from build123d import *

# Parameters (mm, degrees)
SKETCH2_W           = 216
SKETCH2_H           = 193.902
SKETCH2_W_2         = 203.3
SKETCH2_H_2         = 181.202
BOSS_EXTRUDE1_DEPTH = 12.7
SKETCH2_3_W         = 203.3
SKETCH2_3_H         = 181.202
BOSS_EXTRUDE2_DEPTH = 6.35
CUT_EXTRUDE1_DEPTH  = 12.7
SKETCH5_W           = 216
SKETCH5_H           = 193.902
CUT_EXTRUDE2_DEPTH  = 1.27


with BuildPart() as part:
    # Sketch2 → Boss-Extrude1 (new body)
    with BuildSketch(Plane(origin=(0, 0, 0), x_dir=(1, 0, 0), z_dir=(0, 1, 0))):
        with Locations((101.6, 90.551)):
            Rectangle(SKETCH2_W, SKETCH2_H)
        with Locations((101.6, 90.551)):
            Rectangle(SKETCH2_W_2, SKETCH2_H_2, mode=Mode.SUBTRACT)
    extrude(amount=BOSS_EXTRUDE1_DEPTH)

    # Sketch2<3> → Boss-Extrude2 (add)
    with BuildSketch(Plane(origin=(0, 0, 0), x_dir=(1, 0, 0), z_dir=(0, 1, 0))):
        with Locations((101.6, 90.551)):
            Rectangle(SKETCH2_3_W, SKETCH2_3_H)
    extrude(amount=BOSS_EXTRUDE2_DEPTH)

    # Sketch4 → Cut-Extrude1 (cut, symmetric)
    with BuildSketch(Plane(origin=(0, 0, -90.551), x_dir=(-1, 0, 0), z_dir=(0, 0, -1))):
        Polygon((-203.2, 9.645710678), (-204.507721606, 8.337989072), (-204.507721606, 7.018410881), (-203.2, 6.26339746), align=None)
    cut_extrude1 = extrude(amount=CUT_EXTRUDE1_DEPTH, both=True, mode=Mode.SUBTRACT)

    # Sketch5 → Cut-Extrude2 (cut)
    with BuildSketch(Plane(origin=(0, 12.7, 0), x_dir=(1, 0, 0), z_dir=(0, 1, 0))):
        with Locations((101.6, 90.551)):
            Rectangle(SKETCH5_W, SKETCH5_H)
        Polygon((203.2, 77.851), (203.2, 103.251), (203.25, 103.251), (203.25, 181.152), (-0.05, 181.152), (-0.05, -0.05), (203.25, -0.05), (203.25, 77.851), align=None, mode=Mode.SUBTRACT)
    extrude(amount=-CUT_EXTRUDE2_DEPTH, mode=Mode.SUBTRACT)

    # Mirror1: Cut-Extrude1 across plane
    add(cut_extrude1.mirror(Plane.ZY.offset(-101.6)), mode=Mode.SUBTRACT)


solid = part.part
Check sheet for the modelled part. Datum: model origin and axes. Units: mm. A direction names the side the tool comes from. Give positions to 0.01 mm unless a question says otherwise; leave off trailing zeros. Loops run counter-clockwise (first coordinate to the right, second up) from the corner with the lowest first, then second, coordinate; pieces in that order, holes last. Notation, with made-up numbers: M 86.5,3 L 103.5,3 A12 ccw 103.5,23 Z; hole C 22.25,22 d1. An arc over 180 degrees is marked long. Use a Markdown table: item, result. Add a question column.
Q1. Tool access check on faces 4 (the flat face through (100, 6.35, -92)), 5 (the flat face through (209.6, 6, -89)). Record the directions out of +Z, -Z, +X, -X, +Y, -Y that give a thin tool (end or side, any length) a straight path to the whole face; none if there is none.
Q2. Sectioned sample at C-C, the plane z = -93.5. Record the cut outline in (x, y).
Q3. Sectioned sample at A-A, the plane x = 24.5. Record the cut outline in (y, z), then the cut area to 3 significant figures.
Q4. Scan lines: line 1 along X through (y, z) = (9.75, -93.5); line 2 along Z through (x, y) = (85.5, 7.25); line 3 along Y through (x, z) = (190, -117). Record each from-to range of solid material in increasing order. Write a range as [from, to].
Q5. Go/stop test with a flat-tipped pin: pin 1 (3 mm diameter, centred on x = 144, z = -62, fed in from +Y). Record where the tip stops, or that it passes through.
Q6. Mould release check, pull along X, two halves, no side actions. Record for faces 1 (the flat face through (100, 6, 6.4)), 2 (the flat face through (-0.05, 10, -89)), 3 (the flat face through (-6.4, 6, -89)): pulls with the +X half, pulls with the -X half, needs draft (parallel to the pull), parting line crosses it, or undercut.
Q7. Sectioned sample at B-B, the plane z = -151. Record the cut outline in (x, y).
Verdict:
| question | item | result |
|---|---|---|
| 1 | face 4 | +Y |
| 1 | face 5 | +Z, -Z, +X, +Y, -Y |
| 2 | outline | M -6.4,0 L 209.6,0 L 209.6,11.43 L 203.25,11.43 L 203.25,9.6 L 204.51,8.34 L 204.51,7.02 L 203.2,6.26 L 203.2,6.35 L 0,6.35 L 0,6.26 L -1.31,7.02 L -1.31,8.34 L -0.05,9.6 L -0.05,11.43 L -6.4,11.43 Z |
| 3 | outline | M 0,-187.5 L 11.43,-187.5 L 11.43,-181.15 L 6.35,-181.15 L 6.35,0.05 L 11.43,0.05 L 11.43,6.4 L 0,6.4 Z |
| 3 | area | 1,300 mm^2 |
| 4 | line 1 | [-6.4, -0.05], [203.25, 209.6] |
| 4 | line 2 | [-187.5, -181.15], [0.05, 6.4] |
| 4 | line 3 | [0, 6.35] |
| 5 | pin 1 | y = 6.35 |
| 6 | face 1 | needs draft |
| 6 | face 2 | undercut |
| 6 | face 3 | pulls with the -X half |
| 7 | outline | M -6.4,0 L 209.6,0 L 209.6,11.43 L 203.25,11.43 L 203.25,6.35 L -0.05,6.35 L -0.05,11.43 L -6.4,11.43 Z |
